```python
from build123d import *

# Parameters (mm, degrees)
F0_W      = 59
F0_H      = 54
F1_DEPTH  = 5
F2_W      = 5
F2_H      = 54
F3_DEPTH  = 21.25
F4_W      = 42
F4_H      = 42
F5_DEPTH  = 28
F6_R      = 1.6
F6_R_2    = 11.5
F7_DEPTH  = 33.001
F8_R      = 2.1
F9_DEPTH  = 5.001
F10_W     = 23
F10_H     = 15
F11_DEPTH = 21.001
F13_DEPTH = 33
F14_SIZE  = 3
F16_DEPTH = 10.6937211186
F17_R     = 5
F18_R     = 1.6
F19_DEPTH = 8.25
F20_R     = 1.6
F21_DEPTH = 2.5
F22_R     = 2.1
F23_DEPTH = 5


with BuildPart() as f1:
    # F0 (on Top) → F1 (new body)
    with BuildSketch(Plane.XY):
        with Locations((29.5, 27)):
            Rectangle(F0_W, F0_H)
    extrude(amount=F1_DEPTH)

    # F2 (on face) → F3 (join)
    with BuildSketch(Plane.XY.offset(5)):
        with Locations((2.5, 27)):
            Rectangle(F2_W, F2_H)
    extrude(amount=F3_DEPTH)

    # F4 (on face) → F5 (join)
    with BuildSketch(Plane.XY.offset(5)):
        with Locations((38, 33)):
            Rectangle(F4_W, F4_H)
    extrude(amount=F5_DEPTH)

    # F6 (on face) → F7 (cut, through all)
    with BuildSketch(Plane.XY.offset(33)):
        with Locations((22.8, 48.2)):
            Circle(F6_R)
        with Locations((38, 33)):
            Circle(F6_R_2)
        with Locations((53.2, 48.2)):
            Circle(F6_R)
        with Locations((22.8, 17.8)):
            Circle(F6_R)
        with Locations((53.2, 17.8)):
            Circle(F6_R)
    extrude(amount=-F7_DEPTH, mode=Mode.SUBTRACT)

    # F8 (on face) → F9 (cut, through all)
    with BuildSketch(Plane.XY.offset(5)):
        with Locations((37, 5)):
            Circle(F8_R)
        with Locations((51.5, 5)):
            Circle(F8_R)
    extrude(amount=-F9_DEPTH, mode=Mode.SUBTRACT)

    # F10 (on face) → F11 (cut, through all)
    with BuildSketch(Plane(origin=(0, 54, 0), x_dir=(-1, 0, 0), z_dir=(0, 1, 0))):
        with Locations((-38, 22.25)):
            Rectangle(F10_W, F10_H)
    extrude(amount=-F11_DEPTH, mode=Mode.SUBTRACT)

    # F12 (on face) → F13 (cut)
    with BuildSketch(Plane.YZ.offset(59)):
        Polygon((54, 0), (54, 6.5), (35, 6.5), (21, 0), align=None)
    extrude(amount=-F13_DEPTH, mode=Mode.SUBTRACT)

    # F14
    f14_edges = [f1.edges().sort_by_distance(p)[0] for p in [
        (59, 0, 2.5),
        (59, 12, 19),
        (59, 54, 19.75),
    ]]
    chamfer(f14_edges, length=F14_SIZE)

    # F15 (on face) → F16 (cut, through all)
    with BuildSketch(Plane(origin=(0, 54, 0), x_dir=(-1, 0, 0), z_dir=(0, 1, 0))):
        with BuildLine():
            Line((-32.9, 9.385948213), (-32.9031732506, 9.385948213))
            ThreePointArc((-32.9031732506, 9.385948213), (-37.0015866253, 13.6), (-41.1, 9.385948213))
            Line((-41.1, 9.385948213), (-41.1, 6.5))
            Line((-41.1, 6.5), (-32.9, 6.5))
            Line((-32.9, 6.5), (-32.9, 9.385948213))
        make_face()
    extrude(amount=-F16_DEPTH, mode=Mode.SUBTRACT)

    # F17
    f17_edges = [f1.edges().sort_by_distance(p)[0] for p in [
        (0, 27, 0),
    ]]
    fillet(f17_edges, radius=F17_R)

    # F18 (on face) → F19 (cut, through all)
    with BuildSketch(Plane(origin=(0, 0, 6.5), x_dir=(1, 0, 0), z_dir=(0, 0, -1))):
        with Locations((29.8, -48.2)):
            Circle(F18_R)
    extrude(amount=-F19_DEPTH, mode=Mode.SUBTRACT)

    # F20 (on face) → F21 (cut)
    with BuildSketch(Plane.XY.offset(14.75)):
        Polygon((31.4165807537, 45.4), (33.0331615075, 48.2), (31.4165807537, 51), (28.1834192463, 51), (26.5668384925, 48.2), (28.1834192463, 45.4), align=None)
        with Locations((29.8, 48.2)):
            Circle(F20_R, mode=Mode.SUBTRACT)
    extrude(amount=-F21_DEPTH, mode=Mode.SUBTRACT)

    # F22 (on face) → F23 (cut, through all)
    with BuildSketch(Plane(origin=(0, 0, 0), x_dir=(0, -1, 0), z_dir=(-1, 0, 0))):
        with Locations((-49, 20)):
            Circle(F22_R)
        with Locations((-17, 20)):
            Circle(F22_R)
    extrude(amount=-F23_DEPTH, mode=Mode.SUBTRACT)


solid = f1.part
```
Build history of the part. All positions in model axes, mm. A direction names the side the tool comes from. Round coordinates to 2 decimals unless told otherwise and drop trailing zeros. Write each loop counter-clockwise with the first axis right and the second up, starting at its lowest first coordinate (ties: lowest second). Pieces come first, ordered by that corner, then holes. Notation, with made-up numbers: (34.5, -22.75) - (70.5, -22.75) arc R11 cw to (70.5, -5.75) - close; hole circle Ø11 at (88.25, 2). An arc over 180 degrees is marked (long way). Write each question's results on one line, items separated by ' | '. Start each with the question number.
Item 1: Saw through at A-A (z = 20). Write the cut outline in (x, y).
Item 2: Saw through at D-D (y = 39.5). Write the cut outline in (x, z), and give its area (3 significant figures).
Item 3: Drop flat-ended pins along their axis: P1, Ø10, axis at x = 31, z = 25.5, coming from the -Y side; P2, Ø6.5, axis at x = 37, y = 47, coming from the -Z side; P3, Ø1.5, axis at x = 3.5, y = 28, coming from the +Z side. Give the stop position or say it passes through.
Item 4: Mould opens along Y. For faces 1 (the face through (31.2, 49.5, 12.25)), 2 (the face through (14, 21, 5)), 3 (the face through (58, 14, 19)) say: pulls with the +Y half, pulls with the -Y half, needs draft (parallel to the pull), parting line crosses it, or undercut.
Item 5: Saw through at C-C (x = 22.8). Write the cut outline in (y, z).
Item 6: Wall check: L1, parallel to Y at x = 22.8, z = 11.5; L2, parallel to X at y = 33, z = 14; L3, parallel to X at y = 36.5, z = 29. Give the ranges that are in metal, low to high. Write a range as [from, to].
Item 7: Which spindle directions (+Z, -Z, +X, -X, +Y, -Y) get a long thin tool onto all of the face, cutting with end or side? Do faces 4 (the face through (30, 51, 14)), 5 (the face through (28.7, 46.7, 6.5)), 6 (the face through (49.5, 44, 22)), 7 (the face through (17, 33, 19)), 8 (the face through (2.46, 15.87, 21.77)). Say none if no direction does.
Item 8: Saw through at B-B (y = 5). Write the cut outline in (x, z), and give its area (3 significant figures).
Results are:
1) outline: (0, 0) - (5, 0) - (5, 14.9) - (0, 14.9) - close; (0, 19.1) - (5, 19.1) - (5, 46.9) - (0, 46.9) - close; (0, 51.1) - (5, 51.1) - (5, 54) - (0, 54) - close; (17, 12) - (56, 12) - (59, 15) - (59, 51) - (56, 54) - (49.5, 54) - (49.5, 33) arc R11.5 cw to (26.5, 33) - (26.5, 54) - (17, 54) - close; hole circle Ø3.2 at (22.8, 17.8); hole circle Ø3.2 at (22.8, 48.2); hole circle Ø3.2 at (53.2, 17.8); hole circle Ø3.2 at (53.2, 48.2)
2) outline: (0, 5) arc R5 ccw to (5, 0) - (26, 0) - (26, 6.5) - (28.51, 6.5) - (28.51, 14.75) - (26.5, 14.75) - (26.5, 29.75) - (28.51, 29.75) - (28.51, 33) - (17, 33) - (17, 5) - (5, 5) - (5, 26.25) - (0, 26.25) - close; (47.49, 6.5) - (59, 6.5) - (59, 33) - (47.49, 33) - (47.49, 29.75) - (49.5, 29.75) - (49.5, 14.75) - (47.49, 14.75) - close | area: 794 mm²
3) P1: stops at y = 12 | P2: stops at z = 12 | P3: stops at z = 26.25
4) face 1: undercut | face 2: needs draft | face 3: pulls with the -Y half
5) outline: (0, 0) - (16.2, 0) - (16.2, 33) - (12, 33) - (12, 5) - (0, 5) - close; (19.4, 0) - (46.6, 0) - (46.6, 33) - (19.4, 33) - close; (49.8, 0) - (54, 0) - (54, 33) - (49.8, 33) - close
6) L1: y = [12, 16.2], [19.4, 46.6], [49.8, 54] | L2: x = [0, 5], [17, 26.5], [49.5, 59] | L3: x = [17, 26.5], [49.5, 59]
7) face 4: none | face 5: -Z, +X, +Y | face 6: +Y | face 7: +Z, +Y, -Y | face 8: -X
8) outline: (0, 5) arc R5 ccw to (5, 0) - (34.9, 0) - (34.9, 5) - (5, 5) - (5, 26.25) - (0, 26.25) - close; (39.1, 0) - (49.4, 0) - (49.4, 5) - (39.1, 5) - close; (53.6, 0) - (59, 0) - (59, 5) - (53.6, 5) - close | area: 354 mm²
